Input: part model. Units: mm. Frame: model coordinates. Coordinates: 2 decimals unless noted, no trailing zeros. Order: outer loops, then holes, each group sorted by start corner. A loop starts at its lowest first (then second) coordinate and runs counter-clockwise, first axis right, second up. Notation, with made-up numbers: (-23.5, 73) -> (11.5, 73) arc R12 ccw to (11.5, 77) -> close; hole circle Ø7 at (78.25, -23.75). An arc over 180 degrees is marked (long way). Use one line per item in the form item = value. Start each with the question number.
1) Section query A-A on x = 18.5. Output: boundary loops of the cut face in (y, z), then the cut area to 3 significant figures.
2) Ray query, line 1 along Z through (x, y) = (66.5, 4.35); line 2 along Z through (x, y) = (0, 3.9). Return the intervals inside material, ascending.
3) Section query B-B on z = 30. Output: boundary loops of the cut face in (x, y), then the cut area to 3 significant figures.
4) Pin query (flat end, axial travel): pin 1 (1.1 mm diameter, centred on x = -1.5, y = 3, fed in from -Z); pin 2 (1 mm diameter, centred on x = 1, y = 4, fed in from +Z); pin 3 (1.5 mm diameter, centred on x = -1, y = 4, fed in from +Z). Return the tip coordinate at first contact, or that it passes through.
from build123d import *

# Parameters (mm, degrees)
SKETCH1_R           = 3
BOSS_EXTRUDE1_DEPTH = 6


with BuildPart() as part:
    # Sketch1 → Boss-Extrude1 (new body)
    with BuildSketch(Plane(origin=(0, 0, 0), x_dir=(1, 0, 0), z_dir=(0, 1, 0))):
        Polygon((75, -35), (69, -35), (69, -0.661610306), (65, -0.661610306), (65, -1.98375967), (62, -1.98375967), (62, -0.661610306), (57, -0.661610306), (57, 2.538389694), (62, 2.538389694), (62, 4.016764367), (65, 4.016764367), (65, 2.538389694), (69, 2.538389694), (69, 35), (75, 35), (75, 75), (35, 75), (35, 69), (2.538389694, 69), (2.538389694, 65), (4.016764367, 65), (4.016764367, 62), (2.538389694, 62), (2.538389694, 57), (-0.661610306, 57), (-0.661610306, 62), (-1.98375967, 62), (-1.98375967, 65), (-0.661610306, 65), (-0.661610306, 69), (-35, 69), (-35, 75), (-75, 75), (-75, 35), (-69, 35), (-69, 0.661610306), (-65, 0.661610306), (-65, 1.98375967), (-62, 1.98375967), (-62, 0.661610306), (-57, 0.661610306), (-57, -2.538389694), (-62, -2.538389694), (-62, -4.016764367), (-65, -4.016764367), (-65, -2.538389694), (-69, -2.538389694), (-69, -35), (-75, -35), (-75, -75), (-35, -75), (-35, -69), (-0.661610306, -69), (-0.661610306, -65), (-1.98375967, -65), (-1.98375967, -62), (-0.661610306, -62), (-0.661610306, -57), (2.538389694, -57), (2.538389694, -62), (4.016764367, -62), (4.016764367, -65), (2.538389694, -65), (2.538389694, -69), (35, -69), (35, -75), (75, -75), align=None)
        Circle(SKETCH1_R, mode=Mode.SUBTRACT)
    extrude(amount=BOSS_EXTRUDE1_DEPTH)


solid = part.part
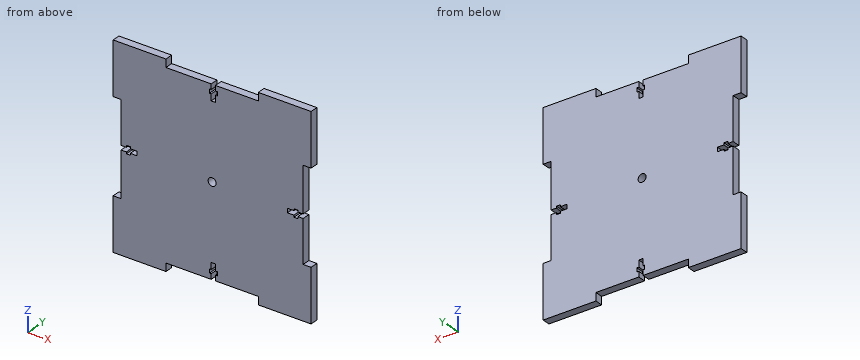
Answers below:
q1.outline = (0, -69) -> (6, -69) -> (6, 69) -> (0, 69) -> close
q1.area = 828 mm^2
q2.line_1 = -75 to -2.54, 0.66 to 75
q2.line_2 = -57 to -3, 3 to 57
q3.outline = (-69, 0) -> (69, 0) -> (69, 6) -> (-69, 6) -> close
q3.area = 828 mm^2
q4.pin_1 = -69
q4.pin_2 = 57
q4.pin_3 = 69
